Read the model definition and answer for the solid it produces. Units are mm, in the model's axes. Face numbers are marked on the shaded views. A direction names the side the tool comes from. Round coordinates to 2 decimals unless told otherwise and drop trailing zeros. Loops run counter-clockwise (first coordinate to the right, second up) from the corner with the lowest first, then second, coordinate; pieces in that order, holes last. Notation, with made-up numbers: M 70.5,61.25 L 121.5,61.25 A23 cw 121.5,81.25 Z; hole C 7,-31 d5. An arc over 180 degrees is marked long. Write each question's results on one line, items separated by ' | '.
from build123d import *

# Parameters (mm, degrees)
BOSS_EXTRUDE1_DEPTH = 152.4
BOSS_EXTRUDE2_DEPTH = 5.08
BOSS_EXTRUDE3_DEPTH = 5.08


with BuildPart() as part:
    # Sketch1 → Boss-Extrude1 (new body)
    with BuildSketch(Plane(origin=(0, 0, 0), x_dir=(1, 0, 0), z_dir=(0, 1, 0))):
        Polygon((-40.411152545, -40.411152545), (-21.87035816, -52.799715283), (0, -57.15), (21.87035816, -52.799715283), (40.411152545, -40.411152545), (52.799715283, -21.87035816), (57.15, 0), (52.799715283, 21.87035816), (40.411152545, 40.411152545), (21.87035816, 52.799715283), (0, 57.15), (-21.87035816, 52.799715283), (-40.411152545, 40.411152545), (-52.799715283, 21.87035816), (-57.15, 0), (-52.799715283, -21.87035816), align=None)
        Polygon((0, 54.61), (-20.898342241, 50.45306127), (-38.615101321, 38.615101321), (-50.45306127, 20.898342241), (-54.61, 0), (-50.45306127, -20.898342241), (-38.615101321, -38.615101321), (-20.898342241, -50.45306127), (0, -54.61), (20.898342241, -50.45306127), (38.615101321, -38.615101321), (50.45306127, -20.898342241), (54.61, 0), (50.45306127, 20.898342241), (38.615101321, 38.615101321), (20.898342241, 50.45306127), align=None, mode=Mode.SUBTRACT)
    extrude(amount=BOSS_EXTRUDE1_DEPTH)

    # Sketch2 → Boss-Extrude2 (add)
    with BuildSketch(Plane(origin=(0, 152.4, 0), x_dir=(1, 0, 0), z_dir=(0, 1, 0))):
        Polygon((-52.799715283, 21.87035816), (-50.45306127, 20.898342241), (-38.615101321, 38.615101321), (-40.411152545, 40.411152545), align=None)
        Polygon((-38.615101321, -38.615101321), (-20.898342241, -50.45306127), (-21.87035816, -52.799715283), (-40.411152545, -40.411152545), align=None)
        Polygon((38.615101321, -38.615101321), (40.411152545, -40.411152545), (52.799715283, -21.87035816), (50.45306127, -20.898342241), align=None)
        Polygon((40.411152545, 40.411152545), (38.615101321, 38.615101321), (20.898342241, 50.45306127), (21.87035816, 52.799715283), align=None)
    extrude(amount=BOSS_EXTRUDE2_DEPTH)

    # Sketch3 → Boss-Extrude3 (add)
    with BuildSketch(Plane.XZ):
        Polygon((38.615101321, -38.615101321), (40.411152545, -40.411152545), (21.87035816, -52.799715283), (20.898342241, -50.45306127), align=None)
        Polygon((50.45306127, 20.898342241), (52.799715283, 21.87035816), (40.411152545, 40.411152545), (38.615101321, 38.615101321), align=None)
        Polygon((-40.411152545, 40.411152545), (-38.615101321, 38.615101321), (-20.898342241, 50.45306127), (-21.87035816, 52.799715283), align=None)
        Polygon((-50.45306127, -20.898342241), (-38.615101321, -38.615101321), (-40.411152545, -40.411152545), (-52.799715283, -21.87035816), align=None)
    extrude(amount=BOSS_EXTRUDE3_DEPTH)


solid = part.part
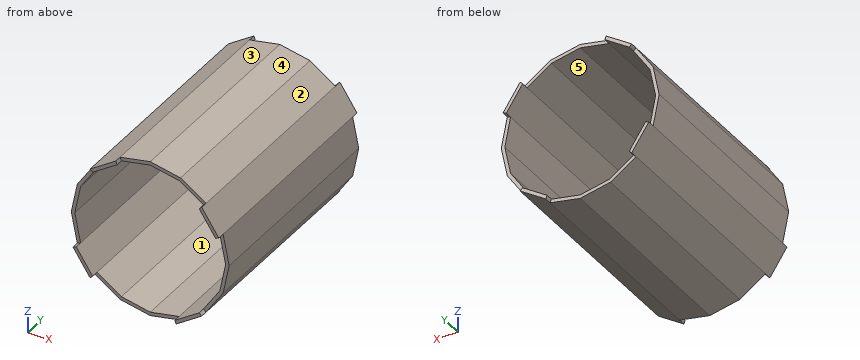
Item 1: For the marked faces 4 and 5, determine the directions among +Z, -Z, +X, -X, +Y, -Y from which every point of the face is accessible in a straight line to the end or side of a thin tool.
Outcome:
face 4: +Z, +X, +Y, -Y | face 5: +Y, -Y
Item 2: The part is cut by section C-C (x = -8). Determine the outline of the cut face in (y, z).
Outcome:
outline: M 0,-55.56 L 152.4,-55.56 L 152.4,-53.02 L 0,-53.02 Z; M 0,53.02 L 152.4,53.02 L 152.4,55.56 L 0,55.56 Z
Item 3: Flat-ended cylindrical pins translate along their axes: pin 1 (5.5 mm diameter, centred on x = 51, z = 1, fed in from +Y); pin 2 (8 mm diameter, centred on y = 91, z = 28, fed in from +X); pin 3 (5.5 mm diameter, centred on x = -52, z = -6, fed in from -Y); pin 4 (4 mm diameter, centred on y = 136.5, z = -13, fed in from +X). Find the tip coordinate at first contact, or state that the pin passes through.
Outcome:
pin 1: passes through | pin 2: stops at x = 51.38 | pin 3: stops at y = 0 | pin 4: stops at x = 54.96
Item 4: The part is cut by section B-B (z = -46). Determine the outline of the cut face in (x, y).
Outcome:
outline: M -32.05,0 L -27.56,0 L -27.56,152.4 L -32.05,152.4 Z; M 27.56,-5.08 L 32.05,-5.08 L 32.05,157.48 L 27.56,157.48 Z
Item 5: Straight lines are drawn through the part: line 1 (Z direction, x = 2, y = 65); line 2 (X direction, y = 147, z = 10); line 3 (X direction, y = 92, z = 18). For each, find the intervals that lie inside material, in ascending order.
Outcome:
line 1: z = -56.75 to -54.21, 54.21 to 56.75 | line 2: x = -55.16 to -52.62, 52.62 to 55.16 | line 3: x = -53.57 to -51.03, 51.03 to 53.57
Item 6: The mould has two halves that part along X. Classify the marked faces 1, 2 and 3: pulls with the +X half, pulls with the -X half, needs draft (parallel to the pull), parting line crosses it, or undercut.
Outcome:
face 1: undercut | face 2: pulls with the +X half | face 3: pulls with the -X half
